Part model, mm, in its own coordinate system. Face numbers are marked on the shaded views. A direction names the side the tool comes from. Round coordinates to 2 decimals unless told otherwise and drop trailing zeros. Write each loop counter-clockwise with the first axis right and the second up, starting at its lowest first coordinate (ties: lowest second). Pieces come first, ordered by that corner, then holes. Notation, with made-up numbers: (36, 20.25) -> (45, 20.25) arc R28 ccw to (45, 51.25) -> close; hole circle Ø9 at (10, -26.5). An arc over 180 degrees is marked (long way). Return JSON: item names as keys, results as strings. Group by question number.
(1) Saw through at A-A (x = 3). List the corners of the cut face in (y, z) (3 decimals), plus the area to 3 significant figures.
(2) Mould opens along Z. For the marked faces 3, 4 and 5 say: +Z half, -Z half, draft (parallel to the pull), parting line (faces both ways), or undercut.
(3) Drill centre lines: L1, parallel to X at y = -1.5, z = -10.5; L2, parallel to Z at x = 1.5, y = -9.5; L3, parallel to Y at x = 9.25, z = -0.5. Where is each one in solid material? Low to high. Write a range as from..to.
(4) Tool access for the marked faces 1 and 2: list every direction of +Z, -Z, +X, -X, +Y, -Y with a clear straight run to the whole face (end or side of a thin tool).
(5) Saw through at B-B (x = 10.75). List the corners of the cut face in (y, z), plus the area to 3 significant figures.
(6) Drop flat-ended pins along their axis: pin 1 Ø4 at (y, z) = (-9, 0) entering from -X; pin 2 Ø2 at (x, z) = (8, -6) entering from -Y; pin 3 Ø4 at (x, z) = (12, 3) entering from -Y. Give the stop position or say it passes through.
from build123d import *

# Parameters (mm, degrees)
F0_R     = 15.875
F1_DEPTH = 15.24
F2_R     = 5.08


with BuildPart() as f1:
    # F0 (on Right) → F1 (new body)
    with BuildSketch(Plane.YZ):
        Circle(F0_R)
    extrude(amount=F1_DEPTH)

    # F2
    f2_edges = [f1.edges().sort_by_distance(p)[0] for p in [
        (15.24, -15.875, 0),
    ]]
    fillet(f2_edges, radius=F2_R)

    # F3 (on Front) → F4 (revolve, cut)
    with BuildSketch(Plane.XZ):
        with BuildLine():
            Line((0, 12.7), (0, 0))
            Line((0, 0), (12.7, 0))
            Line((12.7, 0), (11.43, 2.199705))
            Line((11.43, 2.199705), (11.43, 11.43))
            ThreePointArc((11.43, 11.43), (11.058026, 12.328026), (10.16, 12.7))
            Line((10.16, 12.7), (0, 12.7))
        make_face()
    revolve(axis=Axis((6.35, 0, 0), (1, 0, 0)), mode=Mode.SUBTRACT)


solid = f1.part
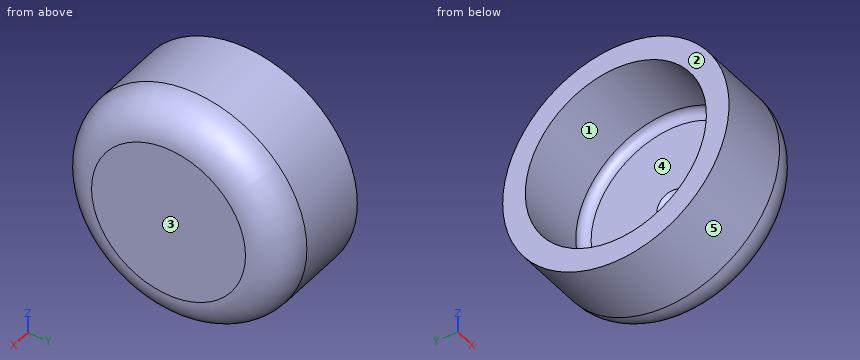
Computed values:
{
 "1": {"outline": "circle Ø31.75 at (0, 0); hole circle Ø25.4 at (0, 0)", "area": "285 mm2"},
 "2": {"face 3": "draft", "face 4": "undercut", "face 5": "parting line"},
 "3": {"L1": "11.43..15.24", "L2": "-12.72..-8.43, 8.43..12.72", "L3": "-15.87..-12.69, 12.69..15.87"},
 "4": {"face 1": "-X", "face 2": "+Z, -Z, -X, +Y, -Y"},
 "5": {"outline": "circle Ø31.68 at (0, 0); hole circle Ø25.11 at (0, 0)", "area": "293 mm2"},
 "6": {"pin 1": "x = 11.43", "pin 2": "y = -15.07", "pin 3": "y = -15.78"}
}
